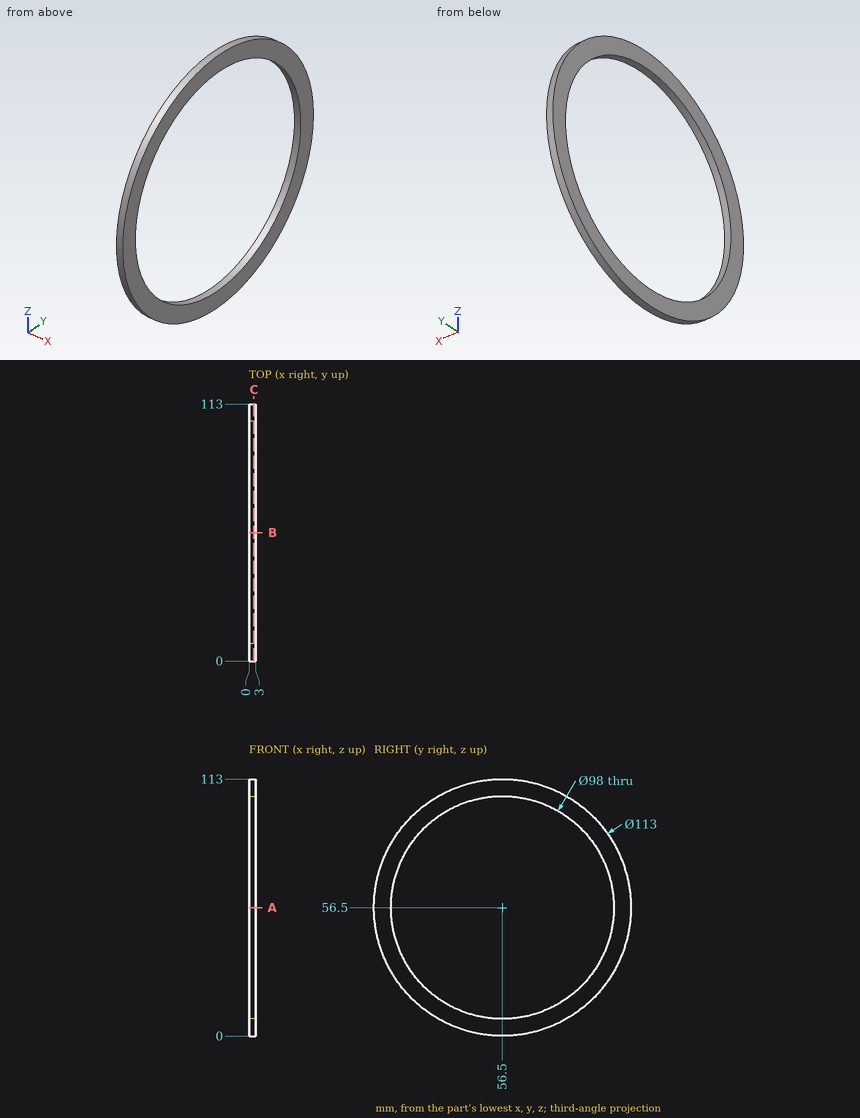
Source: three-view drawing plus pictorial views. Frame: mm from the lowest corner of the part. Coordinates: 2 decimals unless noted, no trailing zeros. Loops run counter-clockwise (first coordinate to the right, second up) from the corner with the lowest first, then second, coordinate; pieces in that order, holes last. Notation, with made-up numbers: (9.25, 35.25) - (42.25, 35.25) arc R27 ccw to (42.25, 53.25) - close; hole circle Ø6 at (-37.5, -1). An arc over 180 degrees is marked (long way). One line per question, with ' | ' between items.
1) Section C-C, the plane x = 2.05. Return loops of the section in (y, z), then the cut area to 3 significant figures.
Report:
outline: circle Ø113 at (56.5, 56.5); hole circle Ø98 at (56.5, 56.5) | area: 2,490 mm²
2) Line query: line 1 along Y through (x, z) = (0.65, 56.5); line 2 along Y through (x, z) = (1.35, 100.5); line 3 along Z through (x, y) = (0.3, 33). Output: solid intervals per line, ascending.
Report:
line 1: y = 0 to 7.5, 105.5 to 113 | line 2: y = 21.06 to 34.94, 78.06 to 91.94 | line 3: z = 5.12 to 13.5, 99.5 to 107.88
3) Section A-A, the plane z = 56.5. Return loops of the section in (x, y).
Report:
outline: (0, 0) - (3, 0) - (3, 7.5) - (0, 7.5) - close; (0, 105.5) - (3, 105.5) - (3, 113) - (0, 113) - close
4) First-contact query: P1, Ø1, axis at x = 2, y = 40, coming from the +Z side; P2, Ø1.5, axis at x = 0.5, z = 66.5, coming from the +Y side; P3, Ø1, axis at x = 2, y = 73.5, coming from the -Z side. Flat tips, straight axial feed; report the tip coordinate or a pass-through.
Report:
P1: stops at z = 110.69 | P2: stops at y = 112.24 | P3: stops at z = 2.46
